from build123d import *

# Parameters (mm, degrees)
BOSS_EXTRUDE1_DEPTH      = 4
BOSS_EXTRUDE1_DEPTH_BACK = 1
SKETCH1_R                = 1.5
CUT_EXTRUDE2_DEPTH       = 122.350119937
BOSS_EXTRUDE2_START      = -5
BOSS_EXTRUDE2_DEPTH      = 3
SKETCH10_R               = 9
SKETCH10_R_2             = 3
CUT_EXTRUDE3_DEPTH       = 3
SKETCH11_R               = 1.886589546
SKETCH11_R_2             = 1
SKETCH11_R_3             = 2
BOSS_EXTRUDE3_DEPTH      = 4
SKETCH12_R               = 1
BOSS_EXTRUDE4_DEPTH      = 1.5


with BuildPart() as part:
    # Sketch1 → Boss-Extrude1 (new, two sides: drawn at the far end of the back side and taken through both)
    with BuildSketch(Plane(origin=(0, 0, 0), x_dir=(0, 0, -1), z_dir=(1, 0, 0)).offset(-BOSS_EXTRUDE1_DEPTH_BACK)):
        Polygon((-75.000724601, -75.086592855), (41.04338169, -75.086592855), (41.04338169, 75.086592855), (-75.000724601, 75.086592855), (-95.199029314, 75.086592855), (-95.199029314, -75.086592855), align=None)
        with Locations((14.384168299, 7.24761685)):
            Circle(SKETCH1_R, mode=Mode.SUBTRACT)
        with Locations((14.384168299, -7.24761685)):
            Circle(SKETCH1_R, mode=Mode.SUBTRACT)
        with BuildLine():
            Line((-55.096951607, 0), (-55.096951607, 2.745063445))
            ThreePointArc((-55.096951607, 2.745063445), (-55.265937152, 3.549666494), (-55.744337674, 4.218303259))
            ThreePointArc((-55.744337674, 4.218303259), (-32.076418352, 64.999999886), (-8.39868917, 4.222124053))
            ThreePointArc((-8.39868917, 4.222124053), (-8.876916854, 3.553557854), (-9.045837474, 2.74910257))
            Line((-9.045837474, 2.74910257), (-9.045837474, 0))
            Line((-9.045837474, 0), (-9.045837474, -2.74910257))
            ThreePointArc((-9.045837474, -2.74910257), (-8.876916854, -3.553557854), (-8.39868917, -4.222124053))
            ThreePointArc((-8.39868917, -4.222124053), (-32.076418352, -64.999999886), (-55.744337674, -4.218303259))
            ThreePointArc((-55.744337674, -4.218303259), (-55.265937152, -3.549666494), (-55.096951607, -2.745063445))
            Line((-55.096951607, -2.745063445), (-55.096951607, 0))
        make_face(mode=Mode.SUBTRACT)
    extrude(amount=BOSS_EXTRUDE1_DEPTH + BOSS_EXTRUDE1_DEPTH_BACK)

    # Sketch8 → Cut-Extrude2 (cut, through all)
    with BuildSketch(Plane(origin=(4, 0, 0), x_dir=(0, 0, -1), z_dir=(1, 0, 0))):
        Polygon((41.04338169, 75.086592855), (41.04338169, 55.086592855), (21.04338169, 75.086592855), align=None)
        Polygon((41.04338169, -75.086592855), (41.04338169, -55.086592855), (21.04338169, -75.086592855), align=None)
        Polygon((-95.199029314, 55.086592855), (-95.199029314, 75.086592855), (-75.199029314, 75.086592855), align=None)
        Polygon((-95.199029314, -55.086592855), (-95.199029314, -75.086592855), (-75.199029314, -75.086592855), align=None)
    extrude(amount=-CUT_EXTRUDE2_DEPTH, mode=Mode.SUBTRACT)

    # Sketch9 → Boss-Extrude2 (add)
    with BuildSketch(Plane(origin=(4, 0, 0), x_dir=(0, 0, -1), z_dir=(1, 0, 0)).offset(BOSS_EXTRUDE2_START)):
        with BuildLine():
            Line((-55.096951607, 0), (-55.096951607, 2.745063445))
            ThreePointArc((-55.096951607, 2.745063445), (-55.265937152, 3.549666494), (-55.744337674, 4.218303259))
            ThreePointArc((-55.744337674, 4.218303259), (-32.076418352, 64.999999886), (-8.39868917, 4.222124053))
            ThreePointArc((-8.39868917, 4.222124053), (-8.876916854, 3.553557854), (-9.045837474, 2.74910257))
            Line((-9.045837474, 2.74910257), (-9.045837474, 0))
            Line((-9.045837474, 0), (-9.045837474, -2.74910257))
            ThreePointArc((-9.045837474, -2.74910257), (-8.876916854, -3.553557854), (-8.39868917, -4.222124053))
            ThreePointArc((-8.39868917, -4.222124053), (-32.076418352, -64.999999886), (-55.744337674, -4.218303259))
            ThreePointArc((-55.744337674, -4.218303259), (-55.265937152, -3.549666494), (-55.096951607, -2.745063445))
            Line((-55.096951607, -2.745063445), (-55.096951607, 0))
        make_face()
    extrude(amount=BOSS_EXTRUDE2_DEPTH)

    # Sketch10 → Cut-Extrude3 (cut)
    with BuildSketch(Plane(origin=(2, 0, 0), x_dir=(0, 0, -1), z_dir=(1, 0, 0))):
        with Locations((-32.073593851, 30)):
            Circle(SKETCH10_R)
        with Locations((-32.073593851, -30)):
            Circle(SKETCH10_R_2)
    extrude(amount=-CUT_EXTRUDE3_DEPTH, mode=Mode.SUBTRACT)

    # Sketch11 → Boss-Extrude3 (add)
    # profile 1 of 2: a face of its own
    with BuildSketch(Plane(origin=(4, 0, 0), x_dir=(0, 0, -1), z_dir=(1, 0, 0))):
        with Locations(Location((-61.096951607, 0, 0), (0, 0, 180))):
            Circle(SKETCH11_R)
        with Locations((-61.096951607, 0)):
            Circle(SKETCH11_R_2, mode=Mode.SUBTRACT)
    # profile 2 of 2: a face of its own
    with BuildSketch(Plane(origin=(4, 0, 0), x_dir=(0, 0, -1), z_dir=(1, 0, 0))):
        with Locations(Location((-3.045837474, 0, 0), (0, 0, 180))):
            Circle(SKETCH11_R_3)
        with Locations((-3.045837474, 0)):
            Circle(SKETCH11_R_2, mode=Mode.SUBTRACT)
    extrude(amount=BOSS_EXTRUDE3_DEPTH)

    # Sketch12 → Boss-Extrude4 (add)
    with BuildSketch(Plane(origin=(8, 0, 0), x_dir=(0, 0, -1), z_dir=(1, 0, 0))):
        with BuildLine():
            Line((-65.096951607, 0), (-65.096951607, 18.404404175))
            ThreePointArc((-65.096951607, 18.404404175), (-32.080235813, 64.99999937), (0.954162526, 18.416938717))
            Line((0.954162526, 18.416938717), (0.954162526, 0))
            Line((0.954162526, 0), (0.954162526, -18.416938717))
            ThreePointArc((0.954162526, -18.416938717), (-32.080235813, -64.99999937), (-65.096951607, -18.404404175))
            Line((-65.096951607, -18.404404175), (-65.096951607, 0))
        make_face()
        with Locations((-61.096951607, 0)):
            Circle(SKETCH12_R, mode=Mode.SUBTRACT)
        with Locations((-3.045837474, 0)):
            Circle(SKETCH12_R, mode=Mode.SUBTRACT)
    extrude(amount=BOSS_EXTRUDE4_DEPTH)


solid = part.part
Input: part model. Units: mm. Frame: model coordinates. A direction names the side the tool comes from. Coordinates: 2 decimals unless noted, no trailing zeros. Order: outer loops, then holes, each group sorted by start corner. A loop starts at its lowest first (then second) coordinate and runs counter-clockwise, first axis right, second up. Notation, with made-up numbers: M 13.25,-35.5 L 31.25,-35.5 A22 cw 31.25,-11.5 Z; hole C 3,-30.5 d6. An arc over 180 degrees is marked long. Write item = value, one per line. Start each with the question number.
(1) First-contact query: P1, Ø1.2, axis at x = 9, y = 8.5, coming from the +Z side; P2, Ø1, axis at y = 0, z = 3.5, coming from the +X side; P3, Ø1.2, axis at x = 9, y = 1.5, coming from the -Z side. Flat tips, straight axial feed; report the tip coordinate or a pass-through.
(2) Section B-B on y = -37. Output: boundary loops of the cut face in (x, z).
(3) Reachability of faces 1 (the cylindrical face through (8.74, -64.988, 31.145)), 2 (the cylindrical face through (5.972, -0.088, 1.048)), 3 (the cylindrical face through (0.52, 32.7, 23.49)) from +Z, -Z, +X, -X, +Y, -Y: full face, straight path, thin tool, end or side. Return the list, or none.
(4) Section A-A on y = 30. Output: boundary loops of the cut face in (x, z), and give its area (3 significant figures).
(5) Pull-direction query (X, two-part tool) for faces 4 (the flat face through (1.54, 64.95, -31.18)), 5 (the cylindrical face through (2.99, 64.98, 33.25)), 6 (the cylindrical face through (2.99, -64.98, 30.9)), 7 (the flat face through (9.5, 1, 32)); classes: released by +X, released by -X, zero draft, split by the parting line, or undercut.
(6) Line query: line 1 along X through (y, z) = (5.5, 60); line 2 along X through (y, z) = (7.5, 41.5); line 3 along Y through (x, z) = (2.75, 27.5). Output: solid intervals per line, ascending. Write a range as [from, to].
(7) Section C-C on z = 57.5. Output: boundary loops of the cut face in (x, y).
(8) Section D-D on z = -33. Output: boundary loops of the cut face in (x, y), and give its area (3 significant figures).
Result set:
q1.P1 = 65.1
q1.P2 = 4
q1.P3 = -0.95
q2.outline = M -1,-41.04 L 4,-41.04 L 4,-2.22 L 2,-2.22 L 2,66.37 L 4,66.37 L 4,95.2 L -1,95.2 Z; M 8,-2.22 L 9.5,-2.22 L 9.5,66.37 L 8,66.37 Z
q3.face_1 = +X
q3.face_2 = none
q3.face_3 = -X
q4.outline = M -1,-41.04 L 4,-41.04 L 4,-2.93 L 2,-2.93 L 2,23.07 L -1,23.07 Z; M -1,41.07 L 2,41.07 L 2,67.07 L 4,67.07 L 4,95.2 L -1,95.2 Z; M 8,-2.93 L 9.5,-2.93 L 9.5,67.07 L 8,67.07 Z
q4.area = 592 mm²
q5.face_4 = zero draft
q5.face_5 = undercut
q5.face_6 = undercut
q5.face_7 = released by +X
q6.line_1 = [-1, 4], [8, 9.5]
q6.line_2 = [-1, 2], [8, 9.5]
q6.line_3 = [-75.09, -64.7], [64.7, 75.09]
q7.outline = M -1,-75.09 L 4,-75.09 L 4,-54.05 L 2,-54.05 L 2,-5.95 L 4,-5.95 L 4,5.95 L 2,5.95 L 2,54.05 L 4,54.05 L 4,75.09 L -1,75.09 Z; M 8,-54.05 L 9.5,-54.05 L 9.5,54.05 L 8,54.05 Z
q8.outline = M -1,-63.13 L 4,-63.13 L 4,63.13 L -1,63.13 Z
q8.area = 631 mm²
